Could you check a few things on this model? Use its own coordinates, in mm. A direction names the side the tool comes from. Give positions to 0.01 mm unless a question says otherwise; leave off trailing zeros. Write each loop counter-clockwise with the first axis right and the second up, starting at its lowest first coordinate (ties: lowest second). Pieces come first, ordered by that corner, then holes. Notation, with made-up numbers: M 51,24.5 L 104,24.5 A16 ccw 104,35.5 Z; hole C 51.5,-33 d1. An arc over 180 degrees is marked long. Use one line per item in the form item = value.
from build123d import *

# Parameters (mm, degrees)
F1_DEPTH = 3


with BuildPart() as f1:
    # F0 (on Top) → F1 (new body)
    with BuildSketch(Plane.XY):
        Polygon((-21.650635, -87.5), (0, -100), (21.650635, -87.5), (24.650635, -92.696152), (67.951905, -67.696152), (64.951905, -62.5), (86.60254, -50), (86.60254, -25), (92.60254, -25), (92.60254, 25), (86.60254, 25), (86.60254, 50), (64.951905, 62.5), (67.951905, 67.696152), (24.650635, 92.696152), (21.650635, 87.5), (0, 100), (-21.650635, 87.5), (-24.650635, 92.696152), (-67.951905, 67.696152), (-64.951905, 62.5), (-86.60254, 50), (-86.60254, 25), (-92.60254, 25), (-92.60254, -25), (-86.60254, -25), (-86.60254, -50), (-64.951905, -62.5), (-67.951905, -67.696152), (-24.650635, -92.696152), align=None)
    extrude(amount=F1_DEPTH)


solid = f1.part
1) I want a section at C-C, the plane x = 81. Please give me the cut outline in (y, z).
Checked values:
outline = M -53.23,0 L 53.23,0 L 53.23,3 L -53.23,3 Z
2) Thinking about a two-plate mould opening in X: for faces 1 (the flat face through (-1, 1, 3)), 2 (the flat face through (10.98, 93.66, 1.48)), 3 (the flat face through (-46.604, -80.021, 1.479)), 4 (the flat face through (46.604, 80.021, 1.479)), which applies, released by +X, released by -X, zero draft, split by the parting line, or undercut?
Checked values:
face_1 = zero draft
face_2 = undercut
face_3 = released by -X
face_4 = released by +X
3) For pin 1 Ø1.5 at (y, z) = (35.5, 1.5) entering from +X; pin 2 Ø1.5 at (x, z) = (88.5, 1.5) entering from -Y; pin 3 Ø1.5 at (x, z) = (-14.5, 2) entering from -Y, each with a flat end and sliding along its axis, tell me the tip position at first contact or that it passes through.
Checked values:
pin_1 = 86.6
pin_2 = -25
pin_3 = -92.06
4) For faces 5 (the flat face through (-10.98, -93.66, 1.48)), 6 (the flat face through (-10.67, 93.84, 1.48)), 7 (the flat face through (-1, 1, 0)), which set-ups out of +Z, -Z, +X, -X, +Y, -Y let a thin tool reach every point of the face, with its end or its side?
Checked values:
face_5 = +Z, -Z, -Y
face_6 = +Z, -Z, +Y
face_7 = -Z, +X, -X, +Y, -Y
5) If I drill on L1, parallel to X at y = -27, z = 2.2; L2, parallel to X at y = 79, z = 1.95; L3, parallel to Y at x = -33, z = 2.3, over which ranges is the centre line in solid material (lowest first)?
Checked values:
L1 = -86.6 to 86.6
L2 = -48.37 to 48.37
L3 = -87.88 to 87.88
6) I want a section at B-B, the plane x = 33. Please give me the cut outline in (y, z).
Checked values:
outline = M -87.88,0 L 87.88,0 L 87.88,3 L -87.88,3 Z
